from build123d import *

# Parameters (mm, degrees)
CROQUIS1_R              = 7.5
SALIENTE_EXTRUIR1_DEPTH = 20
SALIENTE_EXTRUIR2_DEPTH = 80
CORTAR_EXTRUIR1_DEPTH   = 50
CROQUIS4_R              = 10
CORTAR_EXTRUIR2_DEPTH   = 37


with BuildPart() as part:
    # Croquis1 → Saliente-Extruir1 (new body)
    with BuildSketch(Plane(origin=(0, 0, 0), x_dir=(1, 0, 0), z_dir=(0, 1, 0))):
        with BuildLine():
            Line((6.338028169, 1.369942014), (74.169014085, 16.031365878))
            ThreePointArc((74.169014085, 16.031365878), (86, 30.692789743), (74.169014085, 45.354213607))
            Line((74.169014085, 45.354213607), (6.338028169, 60.015637472))
            ThreePointArc((6.338028169, 60.015637472), (0, 60.692789743), (-6.338028169, 60.015637472))
            Line((-6.338028169, 60.015637472), (-74.169014085, 45.354213607))
            ThreePointArc((-74.169014085, 45.354213607), (-86, 30.692789743), (-74.169014085, 16.031365878))
            Line((-74.169014085, 16.031365878), (-6.338028169, 1.369942014))
            ThreePointArc((-6.338028169, 1.369942014), (0, 0.692789743), (6.338028169, 1.369942014))
        make_face()
        with Locations((-71, 30.692789743)):
            Circle(CROQUIS1_R, mode=Mode.SUBTRACT)
        with Locations((71, 30.692789743)):
            Circle(CROQUIS1_R, mode=Mode.SUBTRACT)
    extrude(amount=SALIENTE_EXTRUIR1_DEPTH)

    # Croquis2 → Saliente-Extruir2 (add)
    with BuildSketch(Plane(origin=(0, 20, 0), x_dir=(1, 0, 0), z_dir=(0, 1, 0))):
        with BuildLine():
            Line((-29.047375097, 23.192789743), (29.047375097, 23.192789743))
            ThreePointArc((29.047375097, 23.192789743), (0, 0.692789743), (-29.047375097, 23.192789743))
        make_face()
        with BuildLine():
            Line((-29.047375097, 38.192789743), (29.047375097, 38.192789743))
            ThreePointArc((29.047375097, 38.192789743), (0, 60.692789743), (-29.047375097, 38.192789743))
        make_face()
    extrude(amount=SALIENTE_EXTRUIR2_DEPTH)

    # Croquis3 → Cortar-Extruir1 (cut)
    with BuildSketch(Plane(origin=(0, 100, 0), x_dir=(1, 0, 0), z_dir=(0, 1, 0))):
        with BuildLine():
            Line((-23.616731357, 49.192789743), (23.616731357, 49.192789743))
            ThreePointArc((23.616731357, 49.192789743), (0, 60.692789743), (-23.616731357, 49.192789743))
        make_face()
        with BuildLine():
            Line((-23.616731357, 12.192789743), (23.616731357, 12.192789743))
            ThreePointArc((23.616731357, 12.192789743), (0, 0.692789743), (-23.616731357, 12.192789743))
        make_face()
    extrude(amount=-CORTAR_EXTRUIR1_DEPTH, mode=Mode.SUBTRACT)

    # Croquis4 → Cortar-Extruir2 (cut)
    with BuildSketch(Plane.XY.offset(-12.192789743)):
        with Locations((0, 76)):
            Circle(CROQUIS4_R)
    extrude(amount=-CORTAR_EXTRUIR2_DEPTH, mode=Mode.SUBTRACT)


solid = part.part
Read the model definition and answer for the solid it produces. Units are mm, in the model's axes. A direction names the side the tool comes from. Round coordinates to 2 decimals unless told otherwise and drop trailing zeros. Write each loop counter-clockwise with the first axis right and the second up, starting at its lowest first coordinate (ties: lowest second). Pieces come first, ordered by that corner, then holes.
1. The part is cut by section C-C, the plane y = 76. Determine the outline of the cut face in (x, z).
2. Given pin 1 Ø17 at (x, z) = (71, -30.69) entering from +Y; pin 2 Ø14 at (x, y) = (-4, 79.5) entering from +Z; pin 3 Ø3.5 at (x, z) = (-11, -8) entering from +Y; pin 4 Ø16 at (x, y) = (0, 76) entering from -Z, each flat-ended and moving along its own axis, determine where each tip first touches the part or whether it passes through.
3. The part is cut by section A-A, the plane x = 0. Determine the outline of the cut face in (y, z).
4. Straight lines are drawn through the part: L1, parallel to Y at x = 0, z = -15.5; L2, parallel to Y at x = 48.5, z = -25; L3, parallel to Z at x = 16, y = 39.5. For each, find the intervals that lie inside material, in ascending order.
5. Which of the six approach directions +Z, -Z, +X, -X, +Y, -Y give full straight-line access (tool end or side, diameter ignored) to faces 4 (the face through (0, 50, -8)), 5 (the face through (-11, 75, -49.193)), 6 (the face through (0, 59, -23.193)), 7 (the face through (-1, 20, -31))?
6. The part is cut by section B-B, the plane y = 52. Determine the outline of the cut face in (x, z).
7. Determine the mould class of faces 1 (the face through (40.73, 9.86, -52.58)), 2 (the face through (-1.302, 85.915, -17.616)), 3 (the face through (-1, 0, -31)) for opening direction Y: pulls with the +Y half, pulls with the -Y half, needs draft (parallel to the pull), parting line crosses it, or undercut.
8. The part is cut by section D-D, the plane z = -43.5. Determine the outline of the cut face in (x, y), then the cut area to 3 significant figures.
Values:
1. outline: (-29.05, -38.19) arc R30 ccw to (-23.62, -49.19) - (-10, -49.19) - (-10, -38.19) - close; (-29.05, -23.19) - (-10, -23.19) - (-10, -12.19) - (-23.62, -12.19) arc R30 ccw to start; (10, -49.19) - (23.62, -49.19) arc R30 ccw to (29.05, -38.19) - (10, -38.19) - close; (10, -23.19) - (29.05, -23.19) arc R30 ccw to (23.62, -12.19) - (10, -12.19) - close
2. pin 1: stops at y = 20
2. pin 2: stops at z = -12.19
2. pin 3: stops at y = 50
2. pin 4: passes through
3. outline: (0, -60.69) - (50, -60.69) - (50, -49.19) - (66, -49.19) - (66, -38.19) - (20, -38.19) - (20, -23.19) - (66, -23.19) - (66, -12.19) - (50, -12.19) - (50, -0.69) - (0, -0.69) - close; (86, -49.19) - (100, -49.19) - (100, -38.19) - (86, -38.19) - close; (86, -23.19) - (100, -23.19) - (100, -12.19) - (86, -12.19) - close
4. L1: y = 0 to 66, 86 to 100
4. L2: y = 0 to 20
4. L3: z = -56.07 to -38.19, -23.19 to -5.32
5. face 4: +Z, +X, -X, +Y
5. face 5: -Z, +X, -X, +Y
5. face 6: +X, -X, +Y
5. face 7: +Y
6. outline: (-29.05, -38.19) arc R30 ccw to (-23.62, -49.19) - (23.62, -49.19) arc R30 ccw to (29.05, -38.19) - close; (-29.05, -23.19) - (29.05, -23.19) arc R30 ccw to (23.62, -12.19) - (-23.62, -12.19) arc R30 ccw to start
7. face 1: needs draft
7. face 2: undercut
7. face 3: pulls with the -Y half
8. outline: (-78.81, 0) - (78.81, 0) - (78.81, 20) - (27.13, 20) - (27.13, 100) - (-27.13, 100) - (-27.13, 20) - (-78.81, 20) - close; hole circle Ø20 at (0, 76)
8. area: 7,180 mm2
